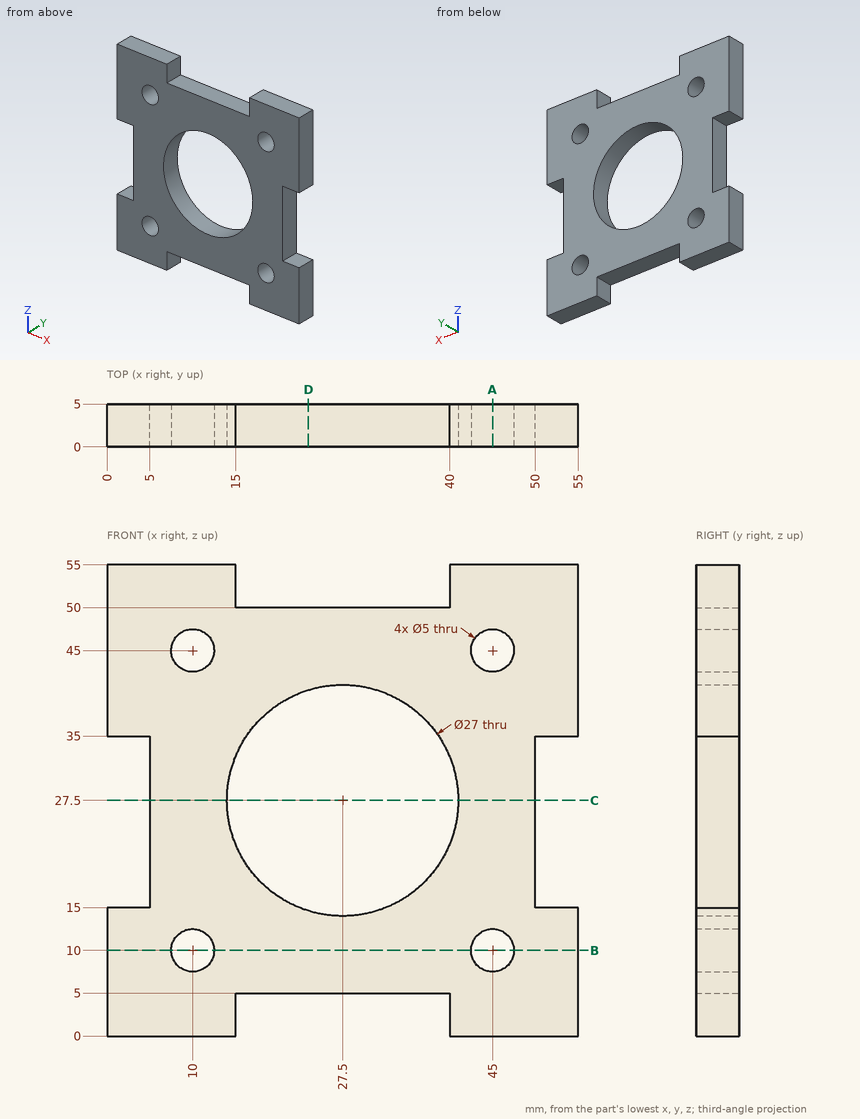
Geometry: see drawing. Coordinates: mm, zero at the bounding-box minimum. Round coordinates to 2 decimals unless told otherwise and drop trailing zeros. Loops run counter-clockwise (first coordinate to the right, second up) from the corner with the lowest first, then second, coordinate; pieces in that order, holes last. Notation, with made-up numbers: M 40.25,64 L 55.25,64 A32 cw 55.25,95 Z; hole C 28,81 d1. An arc over 180 degrees is marked long. Use a Markdown table: item, result. Add a question column.
1. Line query: line 1 (X direction, y = 1.15, z = 10); line 2 (X direction, y = 3.65, z = 27); line 3 (Z direction, x = 46.5, y = 1.8). Output: solid intervals per line, ascending.
2. Contact query for flat-ended pins moving along their axis: P1, Ø2, axis at y = 2, z = 26, coming from the -X side; P2, Ø4.5, axis at x = 10, z = 10, coming from the -Y side; P3, Ø3, axis at x = 24.5, y = 4.5, coming from the -Z side. Output: stop coordinate, or through.
3. Section query A-A on x = 45. Return the cut outline in (y, z), then the cut area to 3 significant figures.
4. Section query B-B on z = 10. Return the cut outline in (x, y), then the cut area to 3 significant figures.
5. Section query C-C on z = 27.5. Return the cut outline in (x, y), then the cut area to 3 significant figures.
6. Section query D-D on x = 23.5. Return the cut outline in (y, z), then the cut area to 3 significant figures.
Reported:
| question | item | result |
|---|---|---|
| 1 | line 1 | x = 0 to 7.5, 12.5 to 42.5, 47.5 to 55 |
| 1 | line 2 | x = 5 to 14.01, 40.99 to 50 |
| 1 | line 3 | z = 0 to 8, 12 to 43, 47 to 55 |
| 2 | P1 | stops at x = 5 |
| 2 | P2 | passes through |
| 2 | P3 | stops at z = 5 |
| 3 | outline | M 0,0 L 5,0 L 5,7.5 L 0,7.5 Z; M 0,12.5 L 5,12.5 L 5,42.5 L 0,42.5 Z; M 0,47.5 L 5,47.5 L 5,55 L 0,55 Z |
| 3 | area | 225 mm² |
| 4 | outline | M 0,0 L 7.5,0 L 7.5,5 L 0,5 Z; M 12.5,0 L 42.5,0 L 42.5,5 L 12.5,5 Z; M 47.5,0 L 55,0 L 55,5 L 47.5,5 Z |
| 4 | area | 225 mm² |
| 5 | outline | M 5,0 L 14,0 L 14,5 L 5,5 Z; M 41,0 L 50,0 L 50,5 L 41,5 Z |
| 5 | area | 90.0 mm² |
| 6 | outline | M 0,5 L 5,5 L 5,14.61 L 0,14.61 Z; M 0,40.39 L 5,40.39 L 5,50 L 0,50 Z |
| 6 | area | 96.1 mm² |
